Read the model definition and answer for the solid it produces. Units are mm, in the model's axes. A direction names the side the tool comes from. Coordinates: 2 decimals unless noted, no trailing zeros. Order: outer loops, then holes, each group sorted by start corner. A loop starts at its lowest first (then second) coordinate and runs counter-clockwise, first axis right, second up. Notation, with made-up numbers: M 63,-23 L 115,-23 A13 ccw 115,-6 Z; hole C 79,81.25 d6. An arc over 180 degrees is marked long. Use a Markdown table: item, result. Add a question column.
1) For faces 1 (the face through (3, -4, 1.85)), 2 (the face through (2, 4, 2)), determine the directions among +Z, -Z, +X, -X, +Y, -Y from which every point of the face is accessible in a straight line to the end or side of a thin tool.
2) Each of these flat-tipped pins is pushed along its axis until it touches: pin 1 Ø1.5 at (x, z) = (-3, 0.5) entering from -Y; pin 2 Ø1 at (x, y) = (2, -5) entering from -Z. Where does it stop, or does it pass through?
3) Find section A-A on x = 0. Write down the section's boundary in (y, z), plus the area to 3 significant figures.
4) Find section C-C on z = 0.55. Write down the section's boundary in (x, y).
5) The mould has two halves that part along X. Classify faces 3 (the face through (-2, 6, -2)), 4 (the face through (3, -4, -1.85)), 5 (the face through (6.466, -2.681, 0.028)): released by +X, released by -X, zero draft, split by the parting line, or undercut.
6) Find the intervals of material crossed by probe 1 along Y at (x, z) = (-0.5, -1.45); probe 2 along Y at (x, z) = (3.25, -0.25); probe 3 along X at (y, z) = (-3, -0.1), in increasing order. Write a range as [from, to].
7) Find section D-D on x = -5.25. Write down the section's boundary in (y, z), plus the area to 3 significant figures.
from build123d import *

# Parameters (mm, degrees)
F0_R     = 6.1
F0_R_2   = 4.7
F1_DEPTH = 1.85
F0_R_3   = 7
F0_R_4   = 4
F2_DEPTH = 2


with BuildPart() as f1:
    # F0 (on Top) → F1 (new body, symmetric)
    with BuildSketch(Plane.XY):
        Circle(F0_R)
        Circle(F0_R_2, mode=Mode.SUBTRACT)
    extrude(amount=F1_DEPTH, both=True)

    # F0 (on Top) → F2 (join, symmetric)
    with BuildSketch(Plane.XY):
        Circle(F0_R_3)
        Circle(F0_R, mode=Mode.SUBTRACT)
        Circle(F0_R_2)
        Circle(F0_R_4, mode=Mode.SUBTRACT)
    extrude(amount=F2_DEPTH, both=True)


solid = f1.part
Check result:
| question | item | result |
|---|---|---|
| 1 | face 1 | +Z |
| 1 | face 2 | +Z, +X, -X, +Y, -Y |
| 2 | pin 1 | stops at y = -6.63 |
| 2 | pin 2 | stops at z = -1.85 |
| 3 | outline | M -7,-2 L -6.1,-2 L -6.1,-1.85 L -4.7,-1.85 L -4.7,-2 L -4,-2 L -4,2 L -4.7,2 L -4.7,1.85 L -6.1,1.85 L -6.1,2 L -7,2 Z; M 4,-2 L 4.7,-2 L 4.7,-1.85 L 6.1,-1.85 L 6.1,-2 L 7,-2 L 7,2 L 6.1,2 L 6.1,1.85 L 4.7,1.85 L 4.7,2 L 4,2 Z |
| 3 | area | 23.2 mm2 |
| 4 | outline | C 0,0 d14; hole C 0,0 d8 |
| 5 | face 3 | zero draft |
| 5 | face 4 | undercut |
| 5 | face 5 | split by the parting line |
| 6 | probe 1 | y = [-6.98, -3.97], [3.97, 6.98] |
| 6 | probe 2 | y = [-6.2, -2.33], [2.33, 6.2] |
| 6 | probe 3 | x = [-6.32, -2.65], [2.65, 6.32] |
| 7 | outline | M -4.63,-2 L -3.11,-2 L -3.11,-1.85 L 3.11,-1.85 L 3.11,-2 L 4.63,-2 L 4.63,2 L 3.11,2 L 3.11,1.85 L -3.11,1.85 L -3.11,2 L -4.63,2 Z |
| 7 | area | 35.2 mm2 |
